The drawing under review shows one solid part. Ordinate dimensions are in mm from its lowest x, y, z. Round coordinates to 2 decimals unless told otherwise and drop trailing zeros. Write each loop counter-clockwise with the first axis right and the second up, starting at its lowest first coordinate (ties: lowest second). Pieces come first, ordered by that corner, then holes. Notation, with made-up numbers: (-37, -36) -> (-3, -36) arc R21 ccw to (-3, -5) -> close; hole circle Ø3 at (-9.75, 36.5). An arc over 180 degrees is marked (long way). Answer in a Markdown table with one row per item. Add a question column.
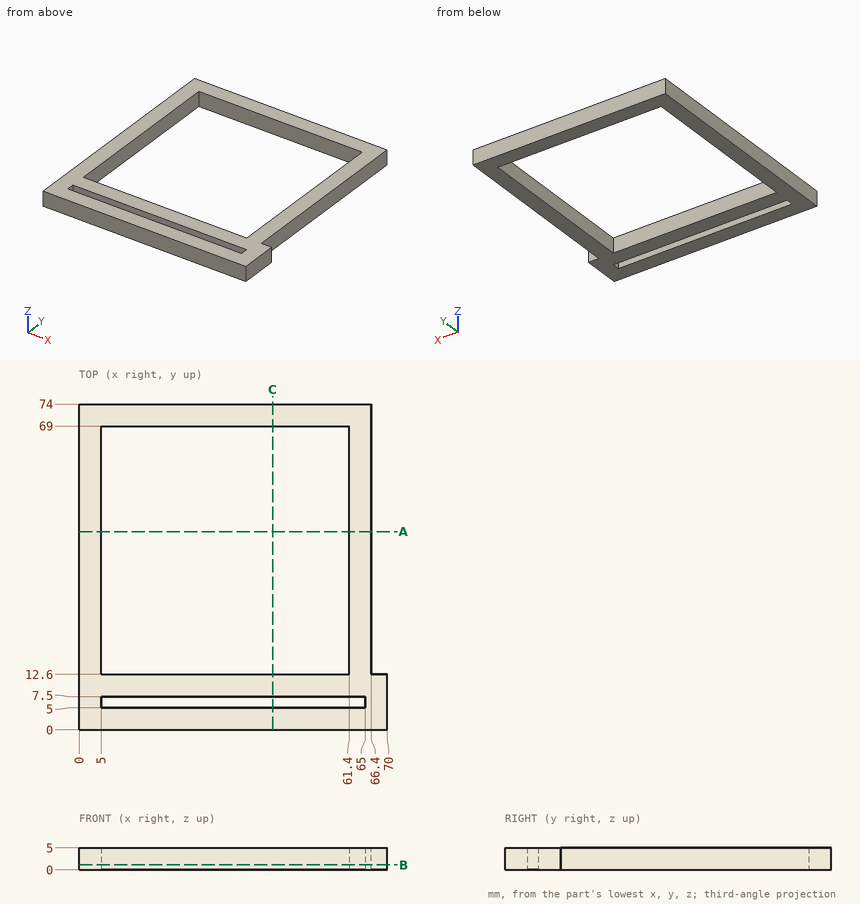
1. For L1, parallel to Y at x = 26, z = 3.1; L2, parallel to X at y = 20, z = 3.95; L3, parallel to X at y = 6.5, z = 2.3, list the stretches that pass through material, from the lowest coordinate up.
2. Add section A-A on y = 45. Write out the cut boundary in (x, z).
3. Insertion check: pin 1 Ø0.8 at (y, z) = (6.5, 3) entering from -X; pin 2 Ø1.8 at (x, z) = (68, 3.5) entering from +Y; pin 3 Ø2.5 at (y, z) = (30.5, 2) entering from +X. Each pin has a flat end and moves straight along its axis. Give the tip position at first contact, or say it passes through.
4. Add section C-C on x = 44. Write out the cut boundary in (y, z).
5. Add section B-B on z = 1.15. Write out the cut boundary in (x, y).
Filled in:
| question | item | result |
|---|---|---|
| 1 | L1 | 0 to 5, 7.5 to 12.6, 69 to 74 |
| 1 | L2 | 0 to 5, 61.4 to 66.4 |
| 1 | L3 | 0 to 5, 65 to 70 |
| 2 | outline | (0, 0) -> (5, 0) -> (5, 5) -> (0, 5) -> close; (61.4, 0) -> (66.4, 0) -> (66.4, 5) -> (61.4, 5) -> close |
| 3 | pin 1 | x = 0 |
| 3 | pin 2 | y = 12.6 |
| 3 | pin 3 | x = 66.4 |
| 4 | outline | (0, 0) -> (5, 0) -> (5, 5) -> (0, 5) -> close; (7.5, 0) -> (12.6, 0) -> (12.6, 5) -> (7.5, 5) -> close; (69, 0) -> (74, 0) -> (74, 5) -> (69, 5) -> close |
| 5 | outline | (0, 0) -> (70, 0) -> (70, 12.6) -> (66.4, 12.6) -> (66.4, 74) -> (0, 74) -> close; hole (5, 5) -> (65, 5) -> (65, 7.5) -> (5, 7.5) -> close; hole (5, 12.6) -> (61.4, 12.6) -> (61.4, 69) -> (5, 69) -> close |
